Source: CAD feature listing. Evaluate the final solid. Frame: model axes, mm. A direction names the side the tool comes from. Round coordinates to 2 decimals unless told otherwise and drop trailing zeros. Order: outer loops, then holes, each group sorted by start corner. A loop starts at its lowest first (then second) coordinate and runs counter-clockwise, first axis right, second up. Notation, with made-up numbers: (14.25, -3) - (55.25, -3) arc R34 ccw to (55.25, 27) - close; hole circle Ø11 at (85.25, 43.5). An arc over 180 degrees is marked (long way). Use one line per item in the form item = value. Start each with the question number.
Q1. Ray query, line 1 (Z direction, x = 1.25, y = 0.75); line 2 (Z direction, x = -3.3, y = 0); line 3 (Z direction, x = -2.75, y = 0). Return the intervals inside material, ascending. Write a range as [from, to].
Q2. Pin query (flat end, axial travel): pin 1 Ø1 at (y, z) = (1, -4.5) entering from +X; pin 2 Ø2.5 at (y, z) = (-1.5, -10.5) entering from -X; pin 3 Ø4 at (y, z) = (0, -12.5) entering from +X. Return the tip coordinate at first contact, or that it passes through.
Q3. Cut plane D-D, the plane z = 8. Return the cut outline in (x, y).
Q4. Cut plane C-C, the plane y = -0.75. Return the cut outline in (x, z), and give its area (3 significant figures).
Q5. Set-up query: faces 4 (the flat face through (1, 0.8, 6.6)), 5 (the flat face through (8, 0, 5)), 6 (the cylindrical face through (4.549, -0.176, 9.339)), 7 (the flat face through (-5, 0, -11)), 8 (the flat face through (2, 0, -8)). Return all of +Z, -Z, +X, -X, +Y, -Y with unobstructed straight access to the full face (end or side cutting, diameter ignored); none if empty.
Q6. Cut plane A-A, the plane x = -3.25. Give the number of separate pieces and of enclosed holes in the cut face, and give its area (3 significant figures).
Q7. Draft query along Z for faces 1 (the cylindrical face through (-4.451, -0.176, 9.339)), 2 (the cylindrical face through (-2.465, -2.859, -15.297)), 3 (the flat face through (-2, 4, -5)). Return one class per face: released by +Z, released by -Z, zero draft, split by the parting line, or undercut.
Q8. Cut plane B-B, the plane z = 4.25. Return the cut outline in (x, y), and give its area (3 significant figures).
from build123d import *

# Parameters (mm, degrees)
F1_DEPTH = 4
F2_R     = 1.35
F3_DEPTH = 25
F4_R     = 1.25
F5_DEPTH = 25
F6_R     = 3.99999


# Not quite as in the source:
# - a fillet or chamfer is up to 0.001 mm smaller than in the source, because OpenCascade refuses the exact size
# - a feature names something its author has since deleted; it is built from what else it names


with BuildPart() as f1:
    # F0 (on Front) → F1 (new body, symmetric)
    with BuildSketch(Plane.XZ):
        with BuildLine():
            ThreePointArc((1, 4.8989794856), (0, -5), (-1, 4.8989794856))
            Line((-1, 4.8989794856), (-1, 11))
            Line((-1, 11), (-8, 11))
            Line((-8, 11), (-8, 0))
            ThreePointArc((-8, 0), (-7.4906334206, -2.8089875327), (-6.0273972603, -5.2602739726))
            ThreePointArc((-6.0273972603, -5.2602739726), (-5.2652950935, -6.53698566), (-5, -8))
            Line((-5, -8), (-5, -16.5))
            Line((-5, -16.5), (0, -16.5))
            Line((0, -16.5), (0, -8))
            Line((0, -8), (5, -8))
            ThreePointArc((5, -8), (5.2652950935, -6.53698566), (6.0273972603, -5.2602739726))
            ThreePointArc((6.0273972603, -5.2602739726), (7.4906334206, -2.8089875327), (8, 0))
            Line((8, 0), (8, 11))
            Line((8, 11), (1, 11))
            Line((1, 11), (1, 4.8989794856))
        make_face()
    extrude(amount=F1_DEPTH, both=True)

    # F2 (on face) → F3 (cut)
    with BuildSketch(Plane.YZ.offset(8)):
        with Locations((0, 8)):
            Circle(F2_R)
    extrude(amount=-F3_DEPTH, mode=Mode.SUBTRACT)

    # F4 (on face) → F5 (cut)
    with BuildSketch(Plane.YZ):
        with Locations((0, -12.5)):
            Circle(F4_R)
    extrude(amount=-F5_DEPTH, mode=Mode.SUBTRACT)

    # F6 (radius 4 in the source; OpenCascade refuses exactly that, so slightly less here)
    f6_edges = [f1.edges().sort_by_distance(p)[0] for p in [
        (-4.5, -4, 11),
        (-4.5, 4, 11),
        (4.5, 4, 11),
        (-2.5, -4, -16.5),
        (-2.5, 4, -16.5),
        (4.5, -4, 11),
    ]]
    fillet(f6_edges, radius=F6_R)


solid = f1.part
Completed:
q1.line_1 = [-8, -4.84], [4.84, 6.88], [9.12, 10.93]
q1.line_2 = [-16.5, -13.75], [-11.25, -3.76], [3.76, 6.65], [9.35, 11]
q1.line_3 = [-16.5, -13.75], [-11.25, -4.18], [4.18, 6.65], [9.35, 11]
q2.pin_1 = 6.93
q2.pin_2 = -5
q2.pin_3 = 0
q3.outline = (-8, -3.87) - (-1, -3.87) - (-1, -1.35) - (-8, -1.35) - close; (-8, 1.35) - (-1, 1.35) - (-1, 3.87) - (-8, 3.87) - close; (1, -3.87) - (8, -3.87) - (8, -1.35) - (1, -1.35) - close; (1, 1.35) - (8, 1.35) - (8, 3.87) - (1, 3.87) - close
q4.outline = (-8, 0) arc R8 ccw to (-6.03, -5.26) arc R4.17 cw to (-5, -8) - (-5, -11.5) - (0, -11.5) - (0, -8) - (5, -8) arc R4.17 cw to (6.03, -5.26) arc R8 ccw to (8, 0) - (8, 6.88) - (1, 6.88) - (1, 4.9) arc R5 cw (long way) to (-1, 4.9) - (-1, 6.88) - (-8, 6.88) - close; (-8, 9.12) - (-1, 9.12) - (-1, 10.93) - (-8, 10.93) - close; (-5, -16.43) - (0, -16.43) - (0, -13.5) - (-5, -13.5) - close; (1, 9.12) - (8, 9.12) - (8, 10.93) - (1, 10.93) - close
q4.area = 192 mm2
q5.face_4 = +Z, +Y, -Y
q5.face_5 = +Z, -Z, +X, +Y, -Y
q5.face_6 = +X, -X
q5.face_7 = -Z, -X, +Y, -Y
q5.face_8 = -Z, +X, +Y, -Y
q6.separate_pieces = 2
q6.enclosed_holes = 2
q6.area = 135 mm2
q7.face_1 = undercut
q7.face_2 = released by -Z
q7.face_3 = zero draft
q8.outline = (-8, -4) - (-2.63, -4) - (-2.63, 4) - (-8, 4) - close; (2.63, -4) - (8, -4) - (8, 4) - (2.63, 4) - close
q8.area = 85.9 mm2
